Geometry check sheet. Reference: the model listing, model coordinates, mm. Round coordinates to 2 decimals unless told otherwise and drop trailing zeros. Write each loop counter-clockwise with the first axis right and the second up, starting at its lowest first coordinate (ties: lowest second). Pieces come first, ordered by that corner, then holes. Notation, with made-up numbers: M 80.25,68 L 94.25,68 A18 ccw 94.25,77 Z; hole C 11,16.25 d4. An arc over 180 degrees is marked long. Put each result on its own line as item: value. Start each with the question number.
(1) Section check B-B on x = 16. Record the cut outline in (y, z).
(2) Section check A-A on z = 1.75. Record the cut outline in (x, y), then the cut area to 3 significant figures.
(3) Gauge pin test, flat ends, axial feed: pin 1 (1.5 mm diameter, centred on y = 28, z = 1, fed in from -X); pin 2 (0.9 mm diameter, centred on y = 27.5, z = 2, fed in from +X); pin 3 (1 mm diameter, centred on y = 215.5, z = 2, fed in from -X); pin 4 (1.5 mm diameter, centred on x = 34, z = 0.5, fed in from +Y). Record the tip position at first contact, or that the pin passes through.
(4) Material ranges on probe 1 along X at (y, z) = (195, 1.4); probe 2 along Y at (x, z) = (75, 0.9); probe 3 along Y at (x, z) = (113.5, 1.6), recorded low to high.
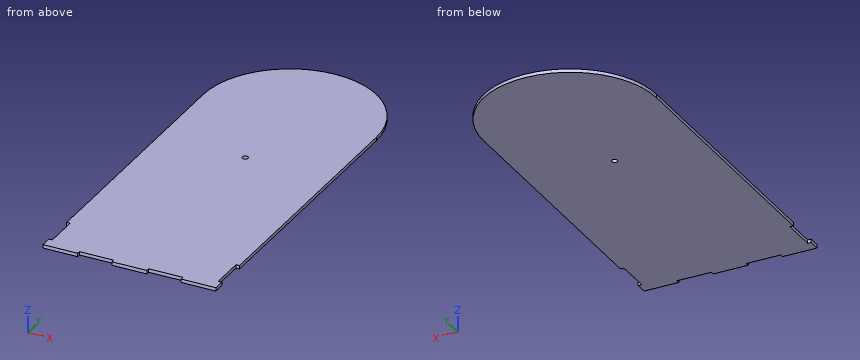
from build123d import *

# Parameters (mm, degrees)
SKETCH1_R           = 2.5
BOSS_EXTRUDE1_DEPTH = 3


with BuildPart() as part:
    # Sketch1 → Boss-Extrude1 (new body)
    with BuildSketch(Plane.XY):
        with BuildLine():
            Line((59.9, 0), (90.1, 0))
            Line((90.1, 0), (90.1, 3))
            Line((90.1, 3), (119.9, 3))
            Line((119.9, 3), (119.9, 0))
            Line((119.9, 0), (150, 0))
            Line((150, 0), (150, 10))
            Line((150, 10), (147, 10))
            Line((147, 10), (147, 39.8))
            Line((147, 39.8), (150, 39.8))
            Line((150, 39.8), (150, 270))
            ThreePointArc((150, 270), (75, 345), (0, 270))
            Line((0, 270), (0, 39.8))
            Line((0, 39.8), (3, 39.8))
            Line((3, 39.8), (3, 10))
            Line((3, 10), (0, 10))
            Line((0, 10), (0, 0))
            Line((0, 0), (30.1, 0))
            Line((30.1, 0), (30.1, 3))
            Line((30.1, 3), (59.9, 3))
            Line((59.9, 3), (59.9, 0))
        make_face()
        with Locations((75, 195)):
            Circle(SKETCH1_R, mode=Mode.SUBTRACT)
    extrude(amount=BOSS_EXTRUDE1_DEPTH)


solid = part.part
Answers follow:
1. outline: M 0,0 L 316.3,0 L 316.3,3 L 0,3 Z
2. outline: M 0,0 L 30.1,0 L 30.1,3 L 59.9,3 L 59.9,0 L 90.1,0 L 90.1,3 L 119.9,3 L 119.9,0 L 150,0 L 150,10 L 147,10 L 147,39.8 L 150,39.8 L 150,270 A75 ccw 0,270 L 0,39.8 L 3,39.8 L 3,10 L 0,10 Z; hole C 75,195 d5
2. area: 49,000 mm^2
3. pin 1: stops at x = 3
3. pin 2: stops at x = 147
3. pin 3: stops at x = 0
3. pin 4: stops at y = 333.28
4. probe 1: x = 0 to 72.5, 77.5 to 150
4. probe 2: y = 0 to 192.5, 197.5 to 345
4. probe 3: y = 3 to 334.36
